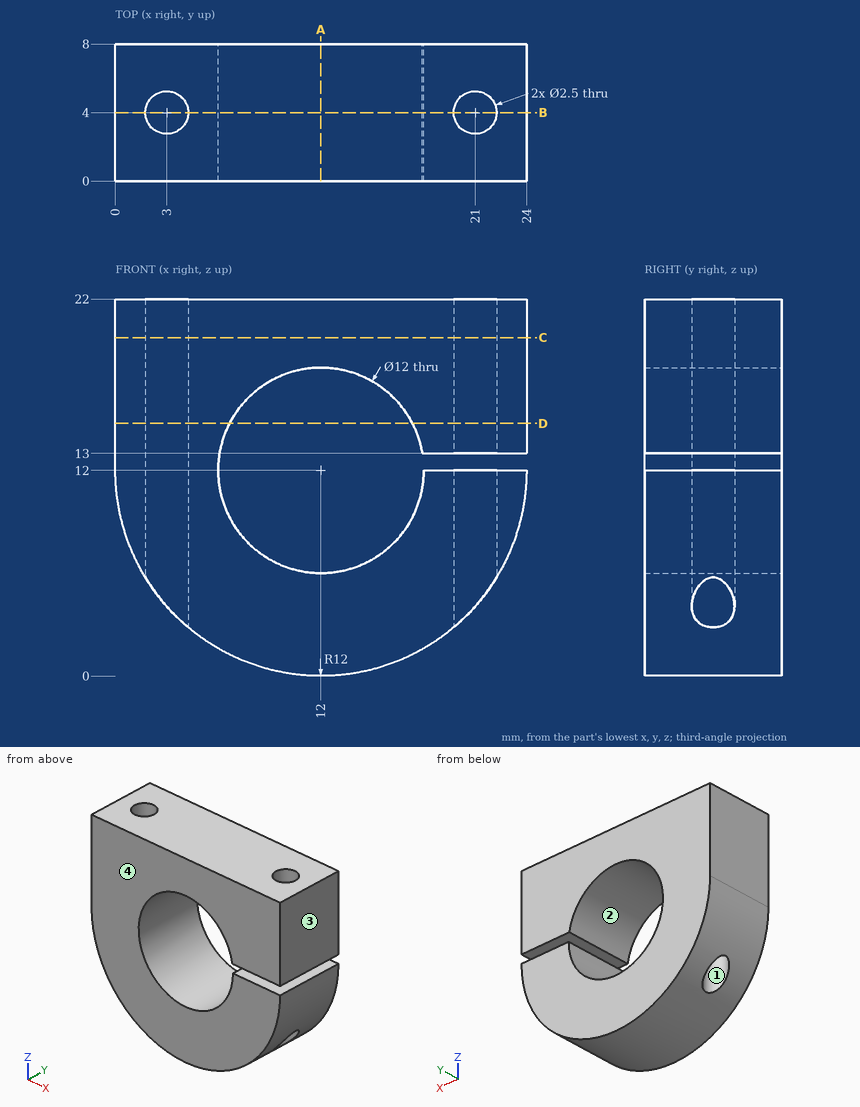
Can you work these out from the drawing? Everything is in mm from the part's minimum corner. Coordinates: 2 decimals unless noted, no trailing zeros. Loops run counter-clockwise (first coordinate to the right, second up) from the corner with the lowest first, then second, coordinate; pieces in that order, holes last. Notation, with made-up numbers: (75, 36) - (113, 36) arc R10 cw to (113, 43) - close; hole circle Ø11 at (60, 16.5). An arc over 180 degrees is marked (long way). Put each result on its own line as item: value. Start each with the question number.
Item 1: Suppose I cut it at C-C (z = 19.75). Please give me the cut outline in (x, y), and give its area (3 significant figures).
Item 2: Suppose I cut it at D-D (z = 14.75). Please give me the cut outline in (x, y), and give its area (3 significant figures).
Item 3: For pin 1 (4 mm diameter, centred on x = 21, y = 4, fed in from -Z); pin 2 (3 mm diameter, centred on x = 21.5, y = 3, fed in from -Z); pin 3 (1.5 mm diameter, centred on x = 21.5, y = 3.5, fed in from -Z), each with a flat end and sliding along its axis, tell me the tip position at first contact or that it passes through.
Item 4: If I drill on line 1 along Y through (x, z) = (21, 19.25); line 2 along X through (y, z) = (4.5, 9); line 3 along Z through (x, y) = (19.75, 2.5), over which ranges is the centre line in solid material (lowest first)?
Item 5: Suppose I cut it at B-B (y = 4). Please give me the cut outline in (x, z).
Item 6: If we mould it in two halves opening along X, with no side actions, what happens to the marked faces 1, 2, 3 and 4? For each: +X half, -X half, draft (parallel to the pull), parting line (faces both ways), or undercut.
Item 7: Suppose I cut it at A-A (x = 12). Please give me the cut outline in (y, z), and give its area (3 significant figures).
Here are the results:
1. outline: (0, 0) - (24, 0) - (24, 8) - (0, 8) - close; hole circle Ø2.5 at (3, 4); hole circle Ø2.5 at (21, 4)
1. area: 182 mm²
2. outline: (0, 0) - (6.67, 0) - (6.67, 8) - (0, 8) - close; (17.33, 0) - (24, 0) - (24, 8) - (17.33, 8) - close; hole circle Ø2.5 at (3, 4); hole circle Ø2.5 at (21, 4)
2. area: 96.9 mm²
3. pin 1: z = 2.25
3. pin 2: z = 3.06
3. pin 3: z = 4.39
4. line 1: 0 to 2.75, 5.25 to 8
4. line 2: 0.38 to 1.85, 4.15 to 6.8, 17.2 to 19.85, 22.15 to 23.62
4. line 3: 2.84 to 12, 13 to 22
5. outline: (0, 12) arc R12 ccw to (1.75, 5.76) - (1.75, 22) - (0, 22) - close; (4.25, 2.84) arc R12 ccw to (19.75, 2.84) - (19.75, 12) - (18, 12) arc R6 cw (long way) to (17.92, 13) - (19.75, 13) - (19.75, 22) - (4.25, 22) - close; (22.25, 5.76) arc R12 ccw to (24, 12) - (22.25, 12) - close; (22.25, 13) - (24, 13) - (24, 22) - (22.25, 22) - close
6. face 1: undercut
6. face 2: undercut
6. face 3: +X half
6. face 4: draft
7. outline: (0, 0) - (8, 0) - (8, 6) - (0, 6) - close; (0, 18) - (8, 18) - (8, 22) - (0, 22) - close
7. area: 80.0 mm²
